Autodesk Inventor part; units mm, degrees
ref_plane "YZ Plane" through (0, 0, 0) normal (1, 0, 0) x (0, 1, 0)
ref_plane "XZ Plane" through (0, 0, 0) normal (0, 1, 0) x (-1, 0, 0)
ref_plane "XY Plane" through (0, 0, 0) normal (0, 0, 1) x (1, 0, 0)
sketch "Sketch1" plane through (0, 0, 0) normal (0, 1, 0) x (-1, 0, 0)
  circle A0 centre (0, 0) radius 100
  line L0 (-76.20071, 31.896636) -> (-108.814125, 31.896636)
  line L1 (-108.814125, 31.896636) -> (-108.814125, -31.604509)
  line L2 (-108.814125, -31.604509) -> (-76.20071, -31.604509)
  line L3 (-76.20071, -31.604509) -> (-76.20071, 31.896636)
  point P0 (-94.874417, -31.604509)
  point P1 (-94.776604, 31.896636)
  dimension "d0" = 200
sketch "Sketch1 outline for Extrusion1" plane through (0, 0, 0) normal (0, 1, 0) x (-1, 0, 0)
  line L0 (-94.776604, 31.896636) -> (-108.814125, 31.896636)
  line L1 (-108.814125, 31.896636) -> (-108.814125, -31.604509)
  line L2 (-108.814125, -31.604509) -> (-94.874417, -31.604509)
  arc A0 (-94.874417, -31.604509) -> (-94.776604, 31.896636) centre (0, 0) ccw
extrude "Extrusion1" add sketch "Sketch1 outline for Extrusion1" along normal blind 15.24
sketch "Sketch2" plane through (0, 15.24, 0) normal (0, 1, 0) x (-0.0015403, 0, 0.9999988)
  circle A0 centre (0, 0) radius 69.85
  dimension "d3" = 139.7
sketch "Sketch2 outline for Extrusion2" plane through (0, 15.24, 0) normal (0, 1, 0) x (-0.0015403, 0, 0.9999988)
  circle A0 centre (0, 0) radius 69.85
extrude "Extrusion2" add sketch "Sketch2 outline for Extrusion2" along normal blind 304.8
ref_plane "Work Plane1" through (69.85, 15.24, 0) normal (1, 0, 0) x (0, 0, -1)
sketch "Sketch3" plane through (69.85, 15.24, 0) normal (1, 0, 0) x (0, 0, -1)
  line L0 (-69.85, 0) -> (-69.85, 304.8)
  line L1 (69.85, 304.8) -> (-69.85, 304.8)
  line L2 (-69.85, 174.745803) -> (69.85, 304.8)
  line L3 (69.85, 304.8) -> (-69.85, 304.8)
  line L4 (-69.85, 304.8) -> (-69.85, 174.745803)
  point P0 (0, -15.24)
sketch "Sketch3 outline for Extrusion3" plane through (69.85, 15.24, 0) normal (1, 0, 0) x (0, 0, -1)
  line L0 (-69.85, 174.745803) -> (69.85, 304.8)
  line L1 (-69.85, 304.8) -> (-69.85, 174.745803)
  line L2 (69.85, 304.8) -> (-69.85, 304.8)
extrude "Extrusion3" cut sketch "Sketch3 outline for Extrusion3" against normal through all
shell "Shell1" thickness 2.54 removed faces 1 at (-23.178976, 247.634165, 7.925999)
properties part number "OCAMS"
Design review of the part built by this model. Coordinates are the model's own, in mm. A direction names the side the tool comes from. Give positions to 0.01 mm unless a question says otherwise; leave off trailing zeros. Write each loop counter-clockwise with the first axis right and the second up, starting at its lowest first coordinate (ties: lowest second). Pieces come first, ordered by that corner, then holes. Notation, with made-up numbers: (71.25, 58) -> (121.25, 58) arc R20 ccw to (121.25, 91) -> close; hole circle Ø9 at (-14, 74). An arc over 180 degrees is marked (long way). Answer in a Markdown table with one row per item.
(1) Clearance check with flat-ended pins moving along their axes: pin 1 (6 mm diameter, centred on x = 57, z = 30.5, fed in from +Y); pin 2 (2 mm diameter, centred on y = 44.5, z = -47, fed in from +X); pin 3 (5 mm diameter, centred on x = 45.5, z = -15, fed in from +Y). State where each tip first meets the part, or that it passes through.
Results:
| item | result |
|---|---|
| pin 1 | y = 226.61 |
| pin 2 | x = 52.56 |
| pin 3 | y = 2.54 |
(2) To check wall thickness, follow probe 1 along Z at (x, y) = (-0.5, 186.5); probe 2 along Y at (x, z) = (-43.5, -55); probe 3 along Z at (x, y) = (0, 7.75). State the ranges of each line that lie inside material, in increasing order.
Results:
| item | result |
|---|---|
| probe 1 | -69.85 to -67.31, 67.31 to 69.85 |
| probe 2 | 0 to 2.54, 12.7 to 15.24 |
| probe 3 | -100 to -97.46, 97.46 to 100 |
(3) Consider section B-B (x = 82). State the section outline as (y, z) points, then the cut area to 3 significant figures.
Results:
| item | result |
|---|---|
| outline | (0, -57.24) -> (15.24, -57.24) -> (15.24, 57.24) -> (0, 57.24) -> close; hole (2.54, -52.67) -> (12.7, -52.67) -> (12.7, 52.67) -> (2.54, 52.67) -> close |
| area | 674 mm2 |
(4) For faces 5 (the flat face through (102, 8, 31.897)), 6 (the flat face through (102, 8, -31.605)), 7 (the cylindrical face through (-2.86, 129.49, -67.25)), 8 (the flat face through (100, 8, -29.065)), list the 3-axis set-ups (+Z, -Z, +X, -X, +Y, -Y) from which the entire face can be reached by the end or side of a thin tool; tool diameter is ignored.
Results:
| item | result |
|---|---|
| face 5 | +Z, +X, +Y, -Y |
| face 6 | -Z, +X, +Y, -Y |
| face 7 | +Y |
| face 8 | none |
(5) Consider section C-C (x = -34). State the section outline as (y, z) points, then the cut area to 3 significant figures.
Results:
| item | result |
|---|---|
| outline | (0, -94.04) -> (15.24, -94.04) -> (15.24, -61.02) -> (311.82, -61.02) -> (309.09, -58.09) -> (12.7, -58.09) -> (12.7, -91.34) -> (2.54, -91.34) -> (2.54, 91.34) -> (12.7, 91.34) -> (12.7, 58.09) -> (200.93, 58.09) -> (198.21, 61.02) -> (15.24, 61.02) -> (15.24, 94.04) -> (0, 94.04) -> close |
| area | 2,120 mm2 |
(6) Mouldability with a two-part tool opening along Z and no side actions: class faces 1 (the flat face through (67.59, 249.89, 5.5)), 2 (the cylindrical face through (-97.39, 7.55, 3.72)), 3 (the cylindrical face through (-2.964, 131.641, -69.787)), 4 (the flat face through (-17, 15.24, 68)) as +Z half, -Z half, draft (parallel to the pull), parting line (faces both ways), or undercut.
Results:
| item | result |
|---|---|
| face 1 | +Z half |
| face 2 | undercut |
| face 3 | parting line |
| face 4 | draft |
(7) Consider section A-A (z = 75.5). State the section outline as (x, y) points, then the cut area to 3 significant figures.
Results:
| item | result |
|---|---|
| outline | (-65.57, 0) -> (65.57, 0) -> (65.57, 15.24) -> (-65.57, 15.24) -> close; hole (-61.63, 2.54) -> (61.63, 2.54) -> (61.63, 12.7) -> (-61.63, 12.7) -> close |
| area | 746 mm2 |
(8) Consider section D-D (z = 0). State the section outline as (x, y) points.
Results:
| item | result |
|---|---|
| outline | (-100, 0) -> (108.81, 0) -> (108.81, 15.24) -> (69.85, 15.24) -> (69.85, 255.01) -> (67.31, 255.01) -> (67.31, 12.7) -> (106.27, 12.7) -> (106.27, 2.54) -> (-97.46, 2.54) -> (-97.46, 12.7) -> (-67.31, 12.7) -> (-67.31, 255.01) -> (-69.85, 255.01) -> (-69.85, 15.24) -> (-100, 15.24) -> close |
